Could you check a few things on this drawing? It's one solid part, dimensions in mm from its lowest x, y, z. Give positions to 0.01 mm unless a question says otherwise; leave off trailing zeros. Order: outer loops, then holes, each group sorted by start corner. A loop starts at its lowest first (then second) coordinate and runs counter-clockwise, first axis right, second up.
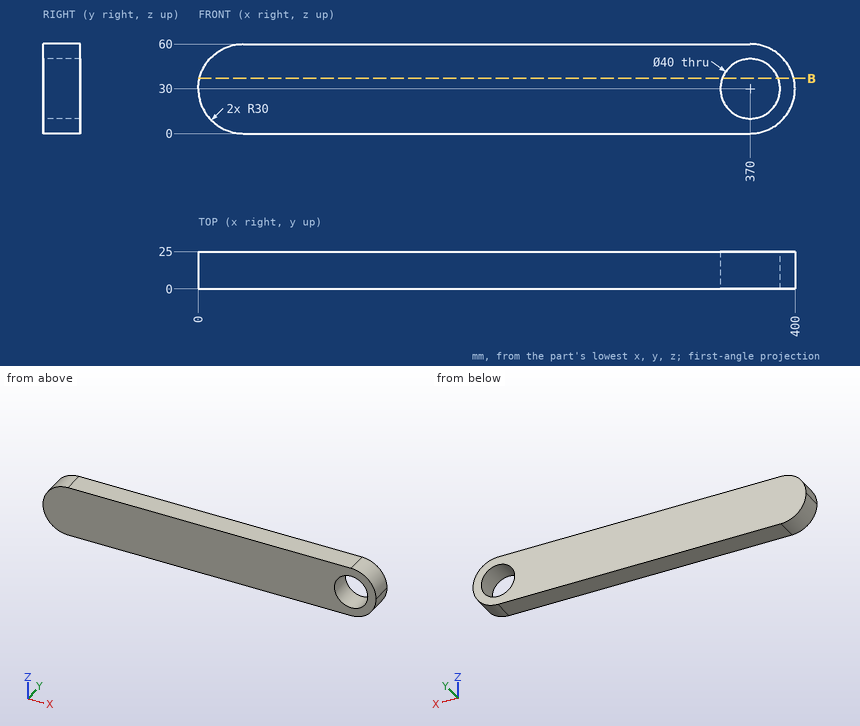
Item 1: For pin 1 (2 mm diameter, centred on y = 14, z = 12.5, fed in from -X) (3 decimals); pin 2 (1.5 mm diameter, centred on y = 18.5, z = 14, fed in from +X); pin 3 (2 mm diameter, centred on y = 13, z = 22, fed in from -X), each with a flat end and sliding along its axis, tell me the tip position at first contact or that it passes through.
Findings:
pin 1: stops at x = 4.945
pin 2: stops at x = 395.83
pin 3: stops at x = 0.83
Item 2: Imagine slicing it at B-B on z = 37. List the corners of the cut face in (x, y) for me (3 decimals).
Findings:
outline: (0.828, 0) - (351.265, 0) - (351.265, 25) - (0.828, 25) - close; (388.735, 0) - (399.172, 0) - (399.172, 25) - (388.735, 25) - close
Item 3: Please list where these lines run through material, in increasing order: line 1 along X through (y, z) = (3, 31.5); line 2 along X through (y, z) = (10.25, 19); line 3 along X through (y, z) = (19.75, 7.5).
Findings:
line 1: x = 0.04 to 350.06, 389.94 to 399.96
line 2: x = 2.09 to 353.3, 386.7 to 397.91
line 3: x = 10.16 to 389.84
